from build123d import *

# Parameters (mm, degrees)
SKETCH_1_R          = 85.5
SKETCH_1_R_2        = 2.65
SKETCH_1_W          = 80
SKETCH_1_H          = 100
EXTRUDE_3_DEPTH     = 10
SKETCH_10_R         = 3.6
SKETCH_10_R_2       = 2.65
CUT_EXTRUDE_2_DEPTH = 10
SKETCH_11_W         = 80
SKETCH_11_H         = 120
CUT_EXTRUDE_3_DEPTH = 10
FILLET_1_R          = 20


with BuildPart() as part:
    # 草图1 → 凸台-拉伸3 (new body)
    with BuildSketch(Plane(origin=(0, 0, 0), x_dir=(1, 0, 0), z_dir=(0, 1, 0))):
        with Locations(Location((0, 0, 0), (0, 0, 270))):
            Circle(SKETCH_1_R)
        with Locations(Location((0, 79, 0), (0, 0, 270))):
            Circle(SKETCH_1_R_2, mode=Mode.SUBTRACT)
        with Locations(Location((55.861435714, 55.861435714, 0), (0, 0, 270))):
            Circle(SKETCH_1_R_2, mode=Mode.SUBTRACT)
        with Locations(Location((79, 0, 0), (0, 0, 270))):
            Circle(SKETCH_1_R_2, mode=Mode.SUBTRACT)
        with Locations(Location((55.861435714, -55.861435714, 0), (0, 0, 270))):
            Circle(SKETCH_1_R_2, mode=Mode.SUBTRACT)
        with Locations(Location((0, -79, 0), (0, 0, 270))):
            Circle(SKETCH_1_R_2, mode=Mode.SUBTRACT)
        with Locations(Location((-55.861435714, -55.861435714, 0), (0, 0, 270))):
            Circle(SKETCH_1_R_2, mode=Mode.SUBTRACT)
        with Locations(Location((-79, 0, 0), (0, 0, 270))):
            Circle(SKETCH_1_R_2, mode=Mode.SUBTRACT)
        with Locations(Location((-55.861435714, 55.861435714, 0), (0, 0, 270))):
            Circle(SKETCH_1_R_2, mode=Mode.SUBTRACT)
        Rectangle(SKETCH_1_W, SKETCH_1_H, mode=Mode.SUBTRACT)
    extrude(amount=EXTRUDE_3_DEPTH)

    # 草图10 → 切除-拉伸2 (cut)
    with BuildSketch(Plane(origin=(0, 10, 0), x_dir=(1, 0, 0), z_dir=(0, 1, 0))):
        with Locations(Location((55, 26.5, 0), (0, 0, 270))):
            Circle(SKETCH_10_R)
        with Locations(Location((65, 0, 0), (0, 0, 270))):
            Circle(SKETCH_10_R_2)
        with Locations(Location((55, -26.5, 0), (0, 0, 270))):
            Circle(SKETCH_10_R)
        with Locations(Location((-55, -26.5, 0), (0, 0, 270))):
            Circle(SKETCH_10_R)
        with Locations(Location((-55, 26.5, 0), (0, 0, 90))):
            Circle(SKETCH_10_R)
        with Locations(Location((-65, 0, 0), (0, 0, 270))):
            Circle(SKETCH_10_R_2)
    extrude(amount=-CUT_EXTRUDE_2_DEPTH, mode=Mode.SUBTRACT)

    # 草图11 → 切除-拉伸3 (cut)
    with BuildSketch(Plane(origin=(0, 10, 0), x_dir=(1, 0, 0), z_dir=(0, 1, 0))):
        Rectangle(SKETCH_11_W, SKETCH_11_H)
    extrude(amount=-CUT_EXTRUDE_3_DEPTH, mode=Mode.SUBTRACT)

    # 圆角1
    fillet_1_edges = [part.edges().sort_by_distance(p)[0] for p in [
        (40, 5, -60),
        (40, 5, 60),
        (-40, 5, 60),
        (-40, 5, -60),
    ]]
    fillet(fillet_1_edges, radius=FILLET_1_R)


solid = part.part
Input: part model. Units: mm. Frame: model coordinates. Coordinates: 2 decimals unless noted, no trailing zeros. Order: outer loops, then holes, each group sorted by start corner. A loop starts at its lowest first (then second) coordinate and runs counter-clockwise, first axis right, second up. Notation, with made-up numbers: M -35,-26.5 L 7,-26.5 A23 ccw 7,9.5 Z; hole C 20,-5.5 d2. An arc over 180 degrees is marked long. One line per question, with ' | ' between items.
Item 1: Pin query (flat end, axial travel): pin 1 (6 mm diameter, centred on x = -20, y = 3.5, fed in from -Z); pin 2 (5 mm diameter, centred on x = -55.86, z = 55.86, fed in from -Y); pin 3 (2 mm diameter, centred on y = 2, z = -13.5, fed in from -X); pin 4 (3 mm diameter, centred on x = 64, y = 6, fed in from +Z). Return the tip coordinate at first contact, or that it passes through.
Geometry results:
pin 1: stops at z = -83.79 | pin 2: passes through | pin 3: stops at x = -84.58 | pin 4: stops at z = 58.34
Item 2: Section A-A (x = 0). Output: boundary loops of the cut face in (y, z).
Geometry results:
outline: M 0,-85.5 L 10,-85.5 L 10,-81.65 L 0,-81.65 Z; M 0,-76.35 L 10,-76.35 L 10,-60 L 0,-60 Z; M 0,60 L 10,60 L 10,76.35 L 0,76.35 Z; M 0,81.65 L 10,81.65 L 10,85.5 L 0,85.5 Z
Item 3: Section B-B (z = -13). Output: boundary loops of the cut face in (x, y), then the cut area to 3 significant figures.
Geometry results:
outline: M -84.51,0 L -40,0 L -40,10 L -84.51,10 Z; M 40,0 L 84.51,0 L 84.51,10 L 40,10 Z | area: 890 mm^2
Item 4: Section C-C (x = 34). Output: boundary loops of the cut face in (y, z), then the cut area to 3 significant figures.
Geometry results:
outline: M 0,-78.45 L 10,-78.45 L 10,-54.28 L 0,-54.28 Z; M 0,54.28 L 10,54.28 L 10,78.45 L 0,78.45 Z | area: 483 mm^2
Item 5: Section D-D (y = 4). Give the number of separate pieces and of enclosed holes in the cut face, then the cut area to 3 significant figures.
Geometry results:
separate pieces: 1 | enclosed holes: 15 | area: 13,300 mm^2
Item 6: Ray query, line 1 along Z through (x, y) = (1, 2.5); line 2 along X through (y, z) = (5.75, -27.5); line 3 along X through (y, z) = (4.25, 26.5). Return the intervals inside material, ascending.
Geometry results:
line 1: z = -85.49 to -81.45, -76.55 to -60, 60 to 76.55, 81.45 to 85.49 | line 2: x = -80.96 to -58.46, -51.54 to -40, 40 to 51.54, 58.46 to 80.96 | line 3: x = -81.29 to -58.6, -51.4 to -40, 40 to 51.4, 58.6 to 81.29
Item 7: Draft query along X for faces 1 (the cylindrical face through (-33.986, 4.93, -54.297)), 2 (the flat face through (-44, 0, 0)), 3 (the cylindrical face through (84.772, 4.93, -11.13)). Return one class per face: released by +X, released by -X, zero draft, split by the parting line, or undercut.
Geometry results:
face 1: undercut | face 2: zero draft | face 3: split by the parting line
